Autodesk Inventor part; units mm, degrees
ref_plane "YZ Plane" through (0, 0, 0) normal (1, 0, 0) x (0, 1, 0)
ref_plane "XZ Plane" through (0, 0, 0) normal (0, 1, 0) x (-1, 0, 0)
ref_plane "XY Plane" through (0, 0, 0) normal (0, 0, 1) x (1, 0, 0)
sketch "Sketch2" plane through (0, 0, 0) normal (0, 0, 1) x (1, 0, 0)
  line L0 (0, 62.5) -> (0, -62.5) construction
  arc A0 (-39.3467, 69.7) -> (39.3467, 69.7) centre (0, 62.5) ccw construction
  arc A1 (61.4792, -51.25) -> (-61.4792, -51.25) centre (0, -62.5) ccw construction
  line L1 (61.4792, -51.25) -> (39.3467, 69.7)
  line L2 (-61.4792, -51.25) -> (-39.3467, 69.7)
  arc A2 (39.3467, 69.7) -> (-39.3467, 69.7) centre (0, 62.5) ccw
  arc A3 (-61.4792, -51.25) -> (61.4792, -51.25) centre (0, -62.5) ccw
  line L3 (0, 62.5) -> (0, 102.5) construction
  point P0 (0, 0)
  point P1 (0, 0)
  dimension "d1" = 125
  dimension "d2" = 80
  dimension "d3" = 125
sketch "Sketch3" plane through (0, 0, 0) normal (1, 0, 0) x (0, 1, 0)
  line L0 (104.9986, 0) -> (98.9986, 0) construction
  line L1 (102.5, 4.25) -> (102.5, -4.25) construction
  line L2 (104.9986, 5.1594) -> (104.9986, -5.1594)
  line L3 (104.9986, -5.1594) -> (98.9986, -2.9756)
  line L4 (98.9986, -2.9756) -> (98.9986, 2.9756)
  line L5 (98.9986, 2.9756) -> (104.9986, 5.1594)
  point P0 (0, 0)
  point P1 (0, 0)
  point P2 (102.5, 0)
  point P3 (102.5, 0)
  point P4 (102.5, 0)
  dimension "d4" = 8.5
  dimension "d5" = 2.4986
  dimension "d6" = 40
  dimension "d7" = 6
sweep "Sweep1" add profiles "Sketch3" path "Sketch2"
equation "\"d4\" = d8"
equation "\"d5\" = d9"
equation "\"d6\" = d10"
equation "\"d7\" = d11"
equation "\"d8\" = 8.5"
equation "\"d9\" = 2.49859"
equation "\"d10\" = 40deg"
equation "\"d11\" = 6"
properties part number "PWTR-0130" material "Rubber"
Here's how the part is built. I have some questions about the finished solid (model axes, mm). A direction names the side the tool comes from. Give positions to 0.01 mm unless a question says otherwise; leave off trailing zeros. Loops run counter-clockwise (first coordinate to the right, second up) from the corner with the lowest first, then second, coordinate; pieces in that order, holes last. Notation, with made-up numbers: (48, 66.25) -> (77, 66.25) arc R21 cw to (77, 101.25) -> close; hole circle Ø2 at (43, 56). An arc over 180 degrees is marked (long way). Use one line per item in the form item = value. Start each with the question number.
1) Please list where these lines run through material, in increasing order: line 1 along X through (y, z) = (-64, -1.5); line 2 along Y through (x, z) = (0, 1.75); line 3 along Y through (x, z) = (-7, 2.75).
2) Imagine slicing it at C-C (z = 1). Please give me the cut outline in (x, y).
3) Imagine slicing it at A-A (x = 0). Please give me the cut outline in (y, z), then the cut area to 3 significant figures.
4) Thinking about a two-plate mould opening in X: for faces 5 (the face through (52.716, 10.521, -0.072)), 6 (the face through (1.456, -121.856, -3.112)), 7 (the face through (0.83, 104.99, 0.07)), which applies, +X half, -X half, draft (parallel to the pull), parting line (faces both ways), or undercut?
5) Imagine slicing it at B-B (y = -62.5). Please give me the cut outline in (x, z), then the cut area to 3 significant figures.
6) For P1, Ø1.5, axis at y = -75, z = -2.5, coming from the +X side; P2, Ø2, axis at y = 66, z = -0.5, coming from the -X side; P3, Ø6, axis at x = -38, y = 61.5, coming from the -Z side, each with a flat end and sliding along its axis, tell me the tip position at first contact or that it passes through.
7) Which directions (+Z, -Z, +X, -X, +Y, -Y) give clear straight access to the entire face, cutting with the end or side of a thin tool? Please do faces 1 (the face through (0.717, 99.367, 3.112)), 2 (the face through (-47.124, 7.748, 0.042)), 3 (the face through (-53.026, 8.828, -0.072)), 4 (the face through (49.72, 9.97, -4.05)).
Check values:
q1.line_1 = -64.98 to -58.98, 58.98 to 64.98
q1.line_2 = -127.5 to -121.5, 99 to 105
q1.line_3 = -127.12 to -121.08, 98.32 to 104.42
q2.outline = (-63.94, -50.8) arc R65 ccw (long way) to (63.94, -50.8) -> (41.8, 70.15) arc R42.5 ccw to (-41.8, 70.15) -> close; hole (-58.03, -51.88) arc R59 ccw (long way) to (58.03, -51.88) -> (35.9, 69.07) arc R36.5 ccw to (-35.9, 69.07) -> close
q3.outline = (-127.5, -5.16) -> (-121.5, -2.98) -> (-121.5, 2.98) -> (-127.5, 5.16) -> close; (99, -2.98) -> (105, -5.16) -> (105, 5.16) -> (99, 2.98) -> close
q3.area = 97.6 mm^2
q4.face_5 = +X half
q4.face_6 = undercut
q4.face_7 = parting line
q5.outline = (-65, -5.16) -> (-59, -2.98) -> (-59, 2.98) -> (-65, 5.16) -> close; (59, -2.98) -> (65, -5.16) -> (65, 5.16) -> (59, 2.98) -> close
q5.area = 97.6 mm^2
q6.P1 = 63.93
q6.P2 = -42.75
q6.P3 = -4.32
q7.face_1 = +Z
q7.face_2 = +Z, -Z
q7.face_3 = +Z, -Z, -X, +Y
q7.face_4 = -Z
